Read the model definition and answer for the solid it produces. Units are mm, in the model's axes. A direction names the side the tool comes from. Coordinates: 2 decimals unless noted, no trailing zeros. Loops run counter-clockwise (first coordinate to the right, second up) from the corner with the lowest first, then second, coordinate; pieces in that order, holes last.
Autodesk Inventor part; units mm, degrees
ref_plane "YZ Plane" through (0, 0, 0) normal (1, 0, 0) x (0, 1, 0)
ref_plane "XZ Plane" through (0, 0, 0) normal (0, 1, 0) x (-1, 0, 0)
ref_plane "XY Plane" through (0, 0, 0) normal (0, 0, 1) x (1, 0, 0)
sketch "Sketch1" plane through (0, 0, 0) normal (0, 0, 1) x (1, 0, 0)
  line L0 (0, 0) -> (28.575, 0)
  line L1 (28.575, 0) -> (28.575, 19.05)
  line L2 (28.575, 19.05) -> (60.325, 19.05)
  line L3 (60.325, 19.05) -> (60.325, 0)
  line L4 (60.325, 0) -> (88.9, 0)
  line L5 (88.9, 0) -> (88.9, 12.7)
  line L6 (88.9, 12.7) -> (69.85, 12.7)
  line L7 (69.85, 12.7) -> (69.85, 63.5)
  line L8 (69.85, 63.5) -> (57.15, 63.5)
  line L9 (57.15, 63.5) -> (57.15, 31.75)
  line L10 (57.15, 31.75) -> (31.75, 31.75)
  line L11 (31.75, 31.75) -> (31.75, 63.5)
  line L12 (31.75, 63.5) -> (19.05, 63.5)
  line L13 (19.05, 63.5) -> (19.05, 12.7)
  line L14 (19.05, 12.7) -> (0, 12.7)
  line L15 (0, 12.7) -> (0, 0)
  dimension "d0" = 19.05
  dimension "d1" = 31.75
  dimension "d2" = 12.7
  dimension "d3" = 25.4
  dimension "d4" = 88.9
  dimension "d5" = 50.8
  dimension "d6" = 19.05
  dimension "d7" = 12.7
extrude "Extrusion1" add sketch "Sketch1" along normal blind 31.75
sketch "Sketch2" plane through (69.85, 12.7, 0) normal (1, 0, 0) x (0, 0, -1)
  point P0 (0, -12.7)
sketch "Sketch3" plane through (69.85, 12.7, 0) normal (1, 0, 0) x (0, 0, -1)
  point P0 (0, -12.7)
sketch "Sketch4" plane through (69.85, 12.7, 0) normal (1, 0, 0) x (0, 0, -1)
  line L0 (0, 0) -> (0, 50.8)
  line L1 (-31.75, 0) -> (-31.75, 50.8)
  arc A0 (0, 47.3352) -> (-31.75, 47.3352) centre (-15.875, 12.7) ccw
  line L2 (0, 50.8) -> (-31.75, 50.8)
  line L3 (-31.75, 47.3352) -> (-31.75, 51.0727)
  line L4 (-31.75, 51.0727) -> (0, 51.0727)
  line L5 (0, 51.0727) -> (0, 47.3352)
  point P0 (0, -12.7)
  dimension "d10" = 38.1
extrude "Extrusion2" cut sketch "Sketch4" against normal through all
sketch "Sketch5" plane through (69.85, 12.7, 31.75) normal (1, 0, 0) x (0, 0, -1)
  circle A0 centre (15.875, 38.1) radius 6.35
  line L0 (31.75, 0) -> (31.75, 47.3352)
  line L1 (31.75, 0) -> (0, 0)
  point P0 (31.75, -12.7)
  dimension "d13" = 12.7
  dimension "d14" = 15.875
  dimension "d15" = 38.1
extrude "Extrusion3" cut sketch "Sketch5" against normal through all
chamfer "Chamfer1" distance 7.62 angle 45 1 edges at (88.9, 6.35, 31.75)
chamfer "Chamfer2" distance 7.62 angle 45 1 edges at (0, 6.35, 31.75)
sketch "Sketch7" plane through (69.85, 12.7, 0) normal (0, 1, 0) x (1, 0, 0)
  circle A0 centre (9.525, -15.875) radius 4.7625
  circle A1 centre (-60.325, -15.875) radius 4.7625
  line L0 (19.05, 0) -> (0, 0)
  line L1 (19.05, 0) -> (19.05, -24.13)
  line L2 (-50.8, 0) -> (-69.85, 0)
  line L3 (-69.85, 0) -> (-69.85, -24.13)
  dimension "d24" = 9.525
  dimension "d25" = 9.525
  dimension "d26" = 15.875
  dimension "d27" = 9.525
  dimension "d28" = 15.875
  dimension "d29" = 9.525
extrude "Extrusion4" cut sketch "Sketch7" against normal through all
equation "\"d0\" = 0.75 * d3"
equation "\"d1\" = 1.25 * d3"
equation "\"d2\" = 0.5 * d3"
equation "\"d4\" = 3.5 * d3"
equation "\"d5\" = 2 * d3"
equation "\"d6\" = 0.75 * d3"
equation "\"d7\" = 0.5 * d3"
equation "\"d25\" = d24"
equation "\"d28\" = d26"
equation "\"d29\" = d27"
properties part number "HW 5 Part 2"
Q1. A cutting plane is placed at C-C (y = 50.8). Give the vertices of the cut face in (x, z) (3 decimals).
Findings below:
outline: (19.05, 0) - (31.75, 0) - (31.75, 9.525) - (19.05, 9.525) - close; (19.05, 22.225) - (31.75, 22.225) - (31.75, 31.75) - (19.05, 31.75) - close; (57.15, 0) - (69.85, 0) - (69.85, 9.525) - (57.15, 9.525) - close; (57.15, 22.225) - (69.85, 22.225) - (69.85, 31.75) - (57.15, 31.75) - close
Q2. A cutting plane is placed at B-B (x = 9). Give the vertices of the cut face in (y, z), then the cut area to 3 significant figures.
Findings below:
outline: (0, 0) - (12.7, 0) - (12.7, 11.14) - (0, 11.14) - close; (0, 20.61) - (12.7, 20.61) - (12.7, 31.75) - (0, 31.75) - close
area: 283 mm2
Q3. Flat-ended cylindrical pins translate along their axes: pin 1 Ø1 at (x, z) = (50, 27) entering from +Y; pin 2 Ø9.5 at (x, z) = (6, 16) entering from +Y; pin 3 Ø15 at (x, z) = (75.5, 16) entering from +Y. Find the tip coordinate at first contact, or state that the pin passes through.
Findings below:
pin 1: stops at y = 31.75
pin 2: stops at y = 12.7
pin 3: stops at y = 63.5
Q4. Determine the mould class of faces 1 (the face through (74.617, 6.439, 15.666)), 2 (the face through (69.85, 38, 16)), 3 (the face through (19.05, 38, 16)), 4 (the face through (17, 0, 16)) for opening direction X: +X half, -X half, draft (parallel to the pull), parting line (faces both ways), or undercut.
Findings below:
face 1: undercut
face 2: +X half
face 3: -X half
face 4: draft
Q5. A cutting plane is placed at A-A (y = 36). Give the vertices of the cut face in (x, z).
Findings below:
outline: (19.05, 0) - (31.75, 0) - (31.75, 31.75) - (19.05, 31.75) - close; (57.15, 0) - (69.85, 0) - (69.85, 31.75) - (57.15, 31.75) - close
Q6. Which of the six approach directions +Z, -Z, +X, -X, +Y, -Y give full straight-line access (tool end or side, diameter ignored) to faces 5 (the face through (44, 24, 0)), 6 (the face through (44, 19.05, 16)), 7 (the face through (14, 12.7, 12)), 8 (the face through (25.489, 57.096, 16.702)), 9 (the face through (31.75, 44, 16))?
Findings below:
face 5: -Z, +X, -X, +Y, -Y
face 6: +Z, -Z, -Y
face 7: +Z, -Z, -X, +Y
face 8: +X, -X
face 9: +Z, -Z, +Y
Q7. A cutting plane is placed at D-D (x = 67). Give the vertices of the cut face in (y, z) (3 decimals), then the cut area to 3 significant figures.
Findings below:
outline: (0, 0) - (60.035, 0) arc R38.1 ccw to (60.035, 31.75) - (0, 31.75) - close; hole circle Ø12.7 at (50.8, 15.875)
area: 1,850 mm2
Q8. Straight lines are drawn through the part: probe 1 along X at (y, z) = (41, 22); probe 2 along X at (y, z) = (26.5, 16.5); probe 3 along Z at (x, y) = (21, 45). For each, find the intervals that lie inside material, in ascending order.
Findings below:
probe 1: x = 19.05 to 31.75, 57.15 to 69.85
probe 2: x = 19.05 to 69.85
probe 3: z = 0 to 13.29, 18.46 to 31.75
